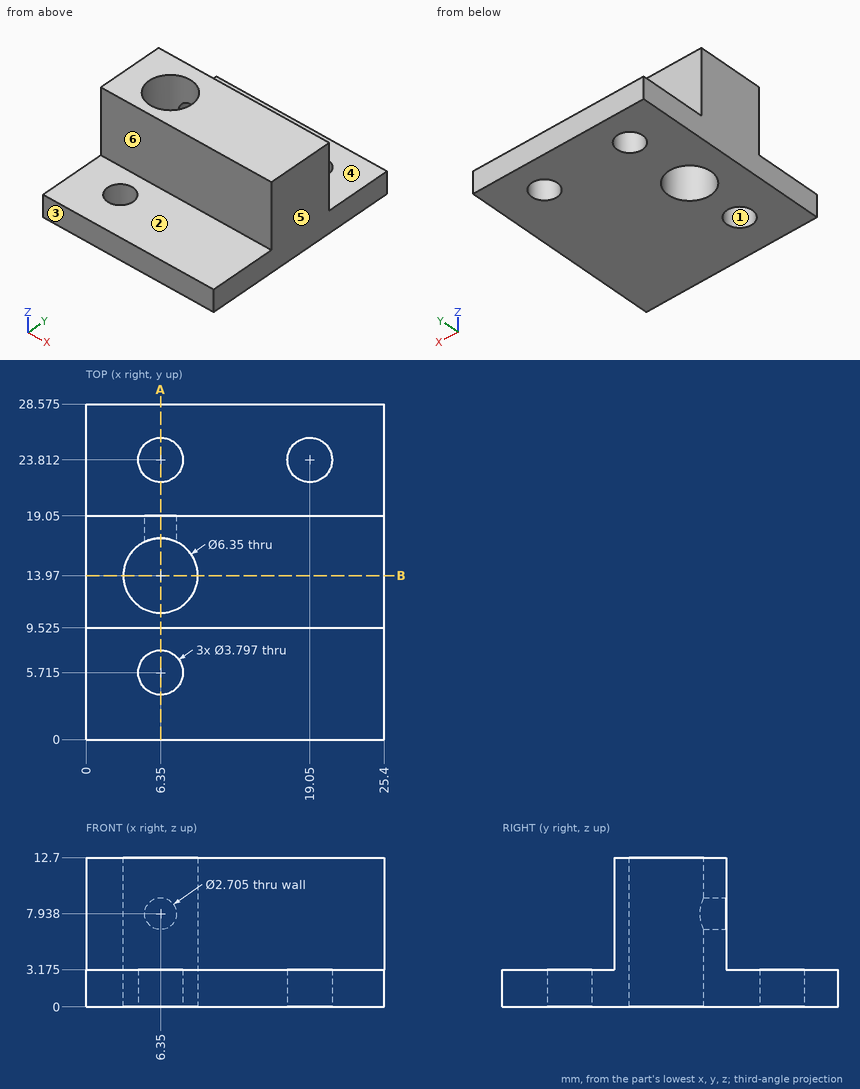
Could you check a few things on this drawing? It's one solid part, dimensions in mm from its lowest x, y, z. A direction names the side the tool comes from. Round coordinates to 2 decimals unless told otherwise and drop trailing zeros. Loops run counter-clockwise (first coordinate to the right, second up) from the corner with the lowest first, then second, coordinate; pieces in that order, holes last. Notation, with made-up numbers: M -14.5,24 L 26.5,24 A16 cw 26.5,49 Z; hole C 37.5,-6 d7. An arc over 180 degrees is marked long. Write each question's results on one line, items separated by ' | '. Start each with the question number.
(1) I want a section at B-B (y = 13.97). Please give me the cut outline in (x, z) (1 decimal), then the cut area to 3 significant figures.
(2) If I drill on probe 1 along X at (y, z) = (24.5, 1); probe 2 along Z at (x, y) = (22.25, 20) (1 decimal); probe 3 along Y at (x, z) = (19.05, 2.25) (1 decimal), over which ranges is the centre line in solid material (lowest first)? Write a range as from..to.
(3) Will these pins go through, and if not, where does the flat tip stop? P1, Ø3, axis at x = 10, y = 23.5, coming from the +Z side (1 decimal); P2, Ø1, axis at x = 23, z = 7, coming from the +Y side; P3, Ø2, axis at x = 6.35, z = 7.94, coming from the -Y side (1 decimal).
(4) On a 3-axis mill with a long thin cutter (end or side, diameter ignored), from which of +Z, -Z, +X, -X, +Y, -Y can I reach the whole of each face in a straight line? I mean the marked faces 4, 5 and 6. Say none if no direction works.
(5) Thinking about a two-plate mould opening in Y: for the marked faces 1, 2 and 3, which applies, pulls with the +Y half, pulls with the -Y half, needs draft (parallel to the pull), parting line crosses it, or undercut?
(6) I want a section at A-A (x = 6.35). State how many separate pieces and enclosed holes the cut face has.
Solved:
1) outline: M 0,0 L 3.2,0 L 3.2,12.7 L 0,12.7 Z; M 9.5,0 L 25.4,0 L 25.4,12.7 L 9.5,12.7 Z | area: 242 mm²
2) probe 1: x = 0..4.58, 8.12..17.28, 20.82..25.4 | probe 2: z = 0..3.2 | probe 3: y = 0..21.9, 25.7..28.6
3) P1: stops at z = 3.2 | P2: stops at y = 19.05 | P3: stops at y = 9.5
4) face 4: +Z, +X, -X, +Y | face 5: +Z, -Z, +X, +Y, -Y | face 6: +Z, +X, -X, -Y
5) face 1: undercut | face 2: needs draft | face 3: pulls with the -Y half
6) separate pieces: 5 | enclosed holes: 0
